The listing builds one solid part. Answer for the finished solid, in the listing's coordinates (mm). Give positions to 0.01 mm unless a question says otherwise; leave off trailing zeros. Write each loop counter-clockwise with the first axis right and the second up, starting at its lowest first coordinate (ties: lowest second). Pieces come first, ordered by that corner, then holes. Notation, with made-up numbers: (-7, -2.5) - (41, -2.5) arc R31 ccw to (41, 26.5) - close; hole circle Ø4 at (16, -10.5). An arc over 180 degrees is marked (long way). Answer in a Markdown table with one row per item. Add a question column.
from build123d import *

# Parameters (mm, degrees)
LOWER_DECK_W        = 101.6
LOWER_DECK_H        = 101.6
LOWER_DECK_R        = 1.9685
LOWER_DECK_R_2      = 27.94
BOSS_EXTRUDE1_DEPTH = 0.8128
FILLET1_R           = 3.81
SKETCH2_W           = 101.6
SKETCH2_H           = 101.6
SKETCH2_R           = 27.94
SKETCH2_R_2         = 1.9685
BOSS_EXTRUDE2_DEPTH = 0.8128
FILLET3_R           = 3.81
BOSS_EXTRUDE3_REACH = 145.87
SKETCH3_R           = 44.45
SKETCH3_R_2         = 27.94


with BuildPart() as part:
    # Lower_Deck → Boss-Extrude1 (new body)
    with BuildSketch(Plane(origin=(0, 0, 0), x_dir=(1, 0, 0), z_dir=(0, 1, 0))):
        with Locations((50.8, 50.8)):
            Rectangle(LOWER_DECK_W, LOWER_DECK_H)
        with Locations(Location((10.3505, 10.3505, 0), (0, 0, 270))):
            Circle(LOWER_DECK_R, mode=Mode.SUBTRACT)
        with Locations(Location((10.3505, 91.2495, 0), (0, 0, 270))):
            Circle(LOWER_DECK_R, mode=Mode.SUBTRACT)
        with Locations(Location((91.2495, 10.3505, 0), (0, 0, 270))):
            Circle(LOWER_DECK_R, mode=Mode.SUBTRACT)
        with Locations(Location((91.2495, 91.2495, 0), (0, 0, 270))):
            Circle(LOWER_DECK_R, mode=Mode.SUBTRACT)
        with Locations(Location((50.8, 50.8, 0), (0, 0, 270))):
            Circle(LOWER_DECK_R_2, mode=Mode.SUBTRACT)
    extrude(amount=BOSS_EXTRUDE1_DEPTH)

    # Fillet1
    fillet1_edges = [part.edges().sort_by_distance(p)[0] for p in [
        (0, 0.4064, -101.6),
        (101.6, 0.4064, -101.6),
        (101.6, 0.4064, 0),
        (0, 0.4064, 0),
    ]]
    fillet(fillet1_edges, radius=FILLET1_R)


with BuildPart() as body_2:
    # Sketch2 → Boss-Extrude2 (new body)
    with BuildSketch(Plane(origin=(0, 7.3152, 0), x_dir=(1, 0, 0), z_dir=(0, 1, 0))):
        with Locations((50.8, 50.8)):
            Rectangle(SKETCH2_W, SKETCH2_H)
        with Locations(Location((50.8, 50.8, 0), (0, 0, 270))):
            Circle(SKETCH2_R, mode=Mode.SUBTRACT)
        with Locations(Location((3.81, 3.81, 0), (0, 0, 270))):
            Circle(SKETCH2_R_2, mode=Mode.SUBTRACT)
        with Locations(Location((3.81, 97.79, 0), (0, 0, 270))):
            Circle(SKETCH2_R_2, mode=Mode.SUBTRACT)
        with Locations(Location((97.79, 97.79, 0), (0, 0, 270))):
            Circle(SKETCH2_R_2, mode=Mode.SUBTRACT)
        with Locations(Location((97.79, 3.81, 0), (0, 0, 270))):
            Circle(SKETCH2_R_2, mode=Mode.SUBTRACT)
    extrude(amount=BOSS_EXTRUDE2_DEPTH)

    # Fillet3
    fillet3_edges = [body_2.edges().sort_by_distance(p)[0] for p in [
        (0, 7.7216, -101.6),
        (101.6, 7.7216, -101.6),
        (101.6, 7.7216, 0),
        (0, 7.7216, 0),
    ]]
    fillet(fillet3_edges, radius=FILLET3_R)

    # Sketch3 → Boss-Extrude3 (add, up to next)
    with BuildSketch(Plane(origin=(0, 0.8128, 0), x_dir=(1, 0, 0), z_dir=(0, 1, 0)), mode=Mode.PRIVATE) as boss_extrude3_sk1:
        with Locations(Location((50.8, 50.8, 0), (0, 0, 90))):
            Circle(SKETCH3_R)
        with Locations(Location((50.8, 50.8, 0), (0, 0, 270))):
            Circle(SKETCH3_R_2, mode=Mode.SUBTRACT)
    boss_extrude3_tool1 = extrude(boss_extrude3_sk1.sketch, amount=BOSS_EXTRUDE3_REACH, mode=Mode.PRIVATE) - body_2.part

    add(part.part)  # Boss-Extrude3 merges part
    add(boss_extrude3_tool1.solids().sort_by_distance((50.8, 0.8128, -7.607236))[0])


solid = body_2.part
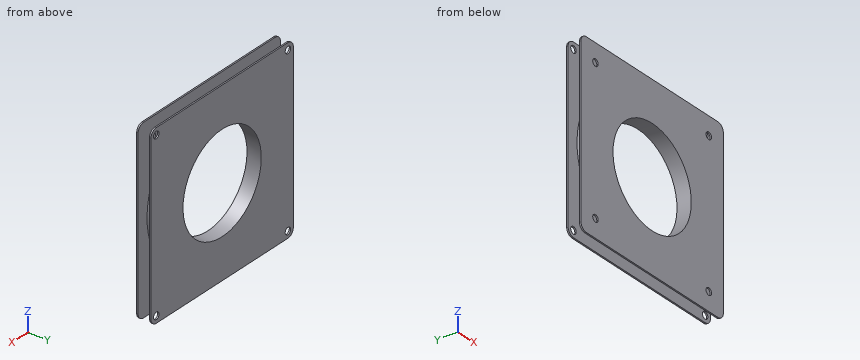
1. Section B-B (z = -63.5) is taken. Give the vertices of the cut face in (x, y).
2. Section D-D (z = -83) is taken. Give the vertices of the cut face in (x, y), and give its area (3 significant figures).
3. Section C-C (y = 3.5) is taken. Give the vertices of the cut face in (x, z).
4. Straight lines are drawn through the part: L1, parallel to Y at x = 72, z = -4.5; L2, parallel to X at y = 2.75, z = -50.8; L3, parallel to Z at x = 61.5, y = 1. For each, find the intervals that lie inside material, in ascending order. Write a range as [from, to].
5. Section A-A (x = 50.8) is taken. Give the vertices of the cut face in (y, z), and give its area (3 significant figures).
6. Given pin 1 Ø2.5 at (x, z) = (3.81, -97.79) entering from +Y; pin 2 Ø2 at (x, y) = (16.5, 2) entering from -Z; pin 3 Ø4 at (y, z) = (4.5, -89.5) entering from +X; pin 4 Ø2 at (x, z) = (61, -75) entering from -Y, each flat-ended and moving along its own axis, determine where each tip first touches the part or whether it passes through.
Geometry check:
| question | item | result |
|---|---|---|
| 1 | outline | (0, 0) - (25.91, 0) - (25.91, 8.13) - (0, 8.13) - (0, 7.32) - (8.2, 7.32) - (8.2, 0.81) - (0, 0.81) - close; (75.69, 0) - (101.6, 0) - (101.6, 0.81) - (93.4, 0.81) - (93.4, 7.32) - (101.6, 7.32) - (101.6, 8.13) - (75.69, 8.13) - close |
| 2 | outline | (0, 0) - (101.6, 0) - (101.6, 0.81) - (81.44, 0.81) - (81.44, 7.32) - (101.6, 7.32) - (101.6, 8.13) - (0, 8.13) - (0, 7.32) - (20.16, 7.32) - (20.16, 0.81) - (0, 0.81) - close |
| 2 | area | 564 mm² |
| 3 | outline | circle Ø88.9 at (50.8, -50.8); hole circle Ø55.88 at (50.8, -50.8) |
| 4 | L1 | [0, 0.81], [7.32, 8.13] |
| 4 | L2 | [6.35, 22.86], [78.74, 95.25] |
| 4 | L3 | [-93.94, -76.61], [-24.99, -7.66] |
| 5 | outline | (0, -101.6) - (0.81, -101.6) - (0.81, -95.25) - (7.32, -95.25) - (7.32, -101.6) - (8.13, -101.6) - (8.13, -78.74) - (0, -78.74) - close; (0, -22.86) - (8.13, -22.86) - (8.13, 0) - (7.32, 0) - (7.32, -6.35) - (0.81, -6.35) - (0.81, 0) - (0, 0) - close |
| 5 | area | 289 mm² |
| 6 | pin 1 | y = 0.81 |
| 6 | pin 2 | z = -80.24 |
| 6 | pin 3 | x = 75.88 |
| 6 | pin 4 | through |
